```python
from build123d import *

# Parameters (mm, degrees)
SKETCH_W     = 44
SKETCH_H     = 46
PAD_DEPTH    = 7
SKETCH001_W  = 25.8
SKETCH001_H  = 25.8
POCKET_DEPTH = 8
SKETCH002_W  = 6.75
SKETCH002_H  = 3
PAD001_DEPTH = 50
SKETCH014_W  = 6.75
SKETCH014_H  = 3.5
PAD014_DEPTH = 50


with BuildPart() as part:
    # Sketch → Pad (new body)
    with BuildSketch(Plane.XY):
        with Locations((-22, -23)):
            Rectangle(SKETCH_W, SKETCH_H)
    extrude(amount=PAD_DEPTH)

    # Sketch001 (on Face6 of Pad) → Pocket (cut)
    with BuildSketch(Plane.XY.offset(7)):
        with Locations((-22, -24.9)):
            Rectangle(SKETCH001_W, SKETCH001_H)
    extrude(amount=-POCKET_DEPTH, mode=Mode.SUBTRACT)

    # Sketch002 (on Face5 of Pocket) → Pad001 (new body)
    with BuildSketch(Plane.XY.offset(7)):
        with Locations((-40.625, -10.5)):
            Rectangle(SKETCH002_W, SKETCH002_H)
    extrude(amount=PAD001_DEPTH)

    # Sketch014 (on Face5 of Pad001) → Pad014 (new body)
    with BuildSketch(Plane.XY.offset(7)):
        with Locations((-40.625, -44.25)):
            Rectangle(SKETCH014_W, SKETCH014_H)
    extrude(amount=PAD014_DEPTH)


solid = part.part
```
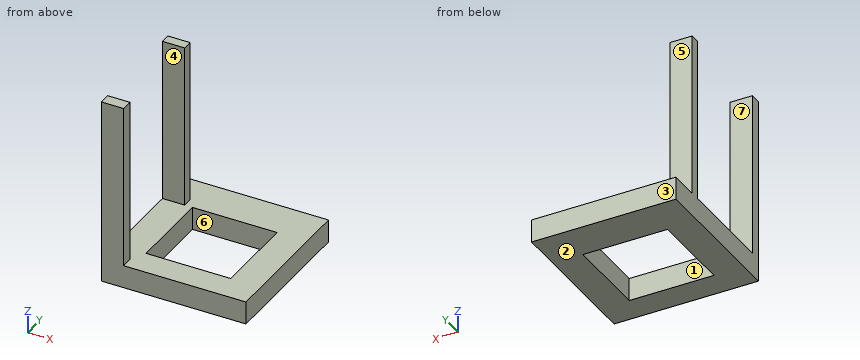
Read the model definition and answer for the solid it produces. Units are mm, in the model's axes. Face numbers are marked on the shaded views. A direction names the side the tool comes from. Coordinates: 2 decimals unless noted, no trailing zeros. Loops run counter-clockwise (first coordinate to the right, second up) from the corner with the lowest first, then second, coordinate; pieces in that order, holes last.
(1) The part is cut by section A-A (z = 19). Determine the outline of the cut face in (x, y).
Solution:
outline: (-44, -46) - (-37.25, -46) - (-37.25, -42.5) - (-44, -42.5) - close; (-44, -12) - (-37.25, -12) - (-37.25, -9) - (-44, -9) - close
(2) Flat-ended cylindrical pins translate along their axes: pin 1 Ø10 at (x, y) = (-14.5, -15) entering from +Z; pin 2 Ø0.9 at (y, z) = (-11, 23) entering from +X; pin 3 Ø5.5 at (x, z) = (-39, 30.5) entering from +Y. Find the tip coordinate at first contact, or state that the pin passes through.
Solution:
pin 1: stops at z = 7
pin 2: stops at x = -37.25
pin 3: stops at y = -9
(3) The part is cut by section B-B (x = -31). Determine the outline of the cut face in (y, z).
Solution:
outline: (-46, 0) - (-37.8, 0) - (-37.8, 7) - (-46, 7) - close; (-12, 0) - (0, 0) - (0, 7) - (-12, 7) - close
(4) A tool of negligible diameter and unlimited length cuts with its end or side. For the marked faces 5, 6 and 7, from which of +Z, -Z, +X, -X, +Y, -Y can it reach the whole face along a straight path? Write none if from no direction.
Solution:
face 5: +Z, +X, -X, +Y
face 6: +Z, -Z
face 7: +Z, +X, -X
(5) The part is cut by section C-C (y = -10.5). Determine the outline of the cut face in (x, z).
Solution:
outline: (-44, 0) - (0, 0) - (0, 7) - (-37.25, 7) - (-37.25, 57) - (-44, 57) - close
(6) Consider line 1 along Y through (x, z) = (-38, 27); line 2 along Y through (x, z) = (-28, 3); line 3 along Z through (x, y) = (-2.5, -2). Determine where each line is inside the solid, lowest interval first.
Solution:
line 1: y = -46 to -42.5, -12 to -9
line 2: y = -46 to -37.8, -12 to 0
line 3: z = 0 to 7
(7) The mould has two halves that part along Y. Classify the marked faces 1, 2, 3 and 4: released by +Y, released by -Y, zero draft, split by the parting line, or undercut.
Solution:
face 1: undercut
face 2: zero draft
face 3: released by +Y
face 4: undercut
(8) The part is cut by section D-D (x = -39). Determine the outline of the cut face in (y, z).
Solution:
outline: (-46, 0) - (0, 0) - (0, 7) - (-9, 7) - (-9, 57) - (-12, 57) - (-12, 7) - (-42.5, 7) - (-42.5, 57) - (-46, 57) - close
